Design review of the part built by this model. Coordinates are the model's own, in mm. A direction names the side the tool comes from. Give positions to 0.01 mm unless a question says otherwise; leave off trailing zeros. Write each loop counter-clockwise with the first axis right and the second up, starting at its lowest first coordinate (ties: lowest second). Pieces come first, ordered by that corner, then holes. Notation, with made-up numbers: (51.5, 7.25) -> (60.5, 7.25) arc R27 cw to (60.5, 37.25) -> close; hole circle Ø1 at (7.5, 10). An arc over 180 degrees is marked (long way). Put each result on its own line as item: value. Start each with the question number.
from build123d import *

# Parameters (mm, degrees)
F0_W     = 2.864896
F0_H     = 4
F1_DEPTH = 10


with BuildPart() as f1:
    # F0 (on Top) → F1 (new body)
    with BuildSketch(Plane.XY):
        with Locations((-36.067552, 27)):
            Rectangle(F0_W, F0_H)
        with Locations((36.067552, 27)):
            Rectangle(F0_W, F0_H)
        Polygon((27.581504, -25), (27.581504, 0), (37.5, 17.196862), (37.5, 25), (34.635104, 25), (31.3, 22), (34.5, 22), (34.5, 18), (25.84857, 3), (24.118284, 0), (24.118284, -22), (-24.118284, -22), (-24.118284, 0), (-25.84857, 3), (-34.5, 18), (-34.5, 22), (-31.3, 22), (-34.635104, 25), (-37.5, 25), (-37.5, 17.196862), (-27.581504, 0), (-27.581504, -25), align=None)
    extrude(amount=F1_DEPTH)


solid = f1.part
Q1. Mouldability with a two-part tool opening along X and no side actions: class faces 1 (the face through (0, -24, 10)), 2 (the face through (-32.6, 8.7, 4.9)), 3 (the face through (34.5, 20, 5)), 4 (the face through (-24.118, -11, 5)) as +X half, -X half, draft (parallel to the pull), parting line (faces both ways), or undercut.
Q2. For pin 1 (2.5 mm diameter, centred on x = -32.5, z = 6, fed in from -Y); pin 2 (1 mm diameter, centred on y = -11, z = 3.5, fed in from -X); pin 3 (1.6 mm diameter, centred on x = 32, z = 3.5, fed in from -Y), all flat-tipped, find the tip position at first contact; note any pin that passes through.
Q3. Take a section at A-A on y = -13.5. Give the boundary of the cut face in (x, z).
Q4. Take a section at B-B on z = 4.75. Give the boundary of the cut face in (x, y).
Q5. To check wall thickness, follow probe 1 along X at (y, z) = (-1, 3); probe 2 along X at (y, z) = (26, 8); probe 3 along Y at (x, z) = (-8, 9.25). State the ranges of each line that lie inside material, in increasing order. Write a range as from..to.
Q6. Take a section at C-C on x = 22. Give the boundary of the cut face in (y, z), then the cut area to 3 significant figures.
Q7. Machinability: for faces 5 (the face through (-33, 22, 5)), 6 (the face through (32.99, 23.52, 4.93)), 7 (the face through (27.582, -13, 5)), which of the approach directions +Z, -Z, +X, -X, +Y, -Y give a long, thin tool a straight path to every point of the face, cutting with its end or side? Answer none if there is none.
Result:
1. face 1: draft
1. face 2: -X half
1. face 3: undercut
1. face 4: undercut
2. pin 1: stops at y = 6.36
2. pin 2: stops at x = -27.58
2. pin 3: stops at y = 6.27
3. outline: (-27.58, 0) -> (-24.12, 0) -> (-24.12, 10) -> (-27.58, 10) -> close; (24.12, 0) -> (27.58, 0) -> (27.58, 10) -> (24.12, 10) -> close
4. outline: (-37.5, 17.2) -> (-27.58, 0) -> (-27.58, -25) -> (27.58, -25) -> (27.58, 0) -> (37.5, 17.2) -> (37.5, 29) -> (34.64, 29) -> (34.64, 25) -> (31.3, 22) -> (34.5, 22) -> (34.5, 18) -> (24.12, 0) -> (24.12, -22) -> (-24.12, -22) -> (-24.12, 0) -> (-34.5, 18) -> (-34.5, 22) -> (-31.3, 22) -> (-34.64, 25) -> (-34.64, 29) -> (-37.5, 29) -> close
5. probe 1: x = -27.58..-24.12, 24.12..27.58
5. probe 2: x = -37.5..-34.64, 34.64..37.5
5. probe 3: y = -25..-22
6. outline: (-25, 0) -> (-22, 0) -> (-22, 10) -> (-25, 10) -> close
6. area: 30.0 mm^2
7. face 5: +Z, -Z
7. face 6: +Z, -Z, +Y
7. face 7: +Z, -Z, +X, -Y
